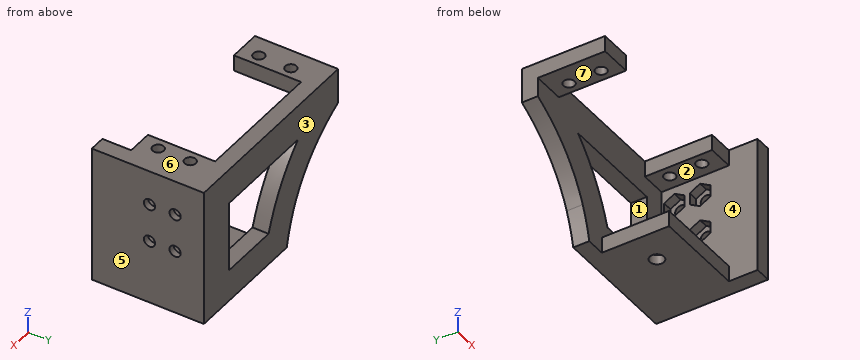
from build123d import *

# Parameters (mm, degrees)
SKETCH1_W                = 10
SKETCH1_H                = 5
BOSS_EXTRUDE1_DEPTH      = 21
BOSS_EXTRUDE1_2_DEPTH    = 21
SKETCH2_W                = 61
SKETCH2_H                = 43
BOSS_EXTRUDE2_DEPTH      = 5
SKETCH3_W                = 30.5
SKETCH3_H                = 5
BOSS_EXTRUDE3_DEPTH      = 21
CUT_EXTRUDE1_REACH       = 74.498
SKETCH4_R                = 2.2
CUT_EXTRUDE2_REACH       = 77.24
SKETCH5_R                = 1.75
CUT_EXTRUDE4_REACH       = 74.231
BOSS_EXTRUDE4_DEPTH      = 3
BOSS_EXTRUDE4_DEPTH_BACK = 2
SKETCH10_W               = 43
SKETCH10_H               = 35
CUT_EXTRUDE5_DEPTH       = 2
CUT_EXTRUDE6_REACH       = 82.077
SKETCH12_R               = 1.75
CUT_EXTRUDE7_DEPTH       = 3


with BuildPart() as part:
    # Sketch1 → Boss-Extrude1 (new body)
    with BuildSketch(Plane(origin=(0, 0, 0), x_dir=(1, 0, 0), z_dir=(0, 1, 0))):
        Rectangle(SKETCH1_W, SKETCH1_H)
    extrude(amount=BOSS_EXTRUDE1_DEPTH)



with BuildPart() as body_2:
    # Sketch1 → Boss-Extrude1 2 (new body)
    with BuildSketch(Plane(origin=(0, 0, 0), x_dir=(1, 0, 0), z_dir=(0, 1, 0))):
        with Locations((51, 0)):
            Rectangle(SKETCH1_W, SKETCH1_H)
    extrude(amount=BOSS_EXTRUDE1_2_DEPTH)


with BuildPart() as part_1:
    add(part.part)

    add(body_2.part)  # Boss-Extrude2 merges body 2
    # Sketch2 → Boss-Extrude2 (add)
    with BuildSketch(Plane(origin=(0, 21, 0), x_dir=(1, 0, 0), z_dir=(0, 1, 0))):
        with Locations((25.5, 19)):
            Rectangle(SKETCH2_W, SKETCH2_H)
    extrude(amount=BOSS_EXTRUDE2_DEPTH)

    # Sketch3 → Boss-Extrude3 (add)
    with BuildSketch(Plane.XZ.offset(-21)):
        with Locations((40.75, -38)):
            Rectangle(SKETCH3_W, SKETCH3_H)
    extrude(amount=BOSS_EXTRUDE3_DEPTH)

    # Sketch4 → Cut-Extrude1 (cut, up to next)
    with BuildSketch(Plane.XY.offset(-35.5), mode=Mode.PRIVATE) as cut_extrude1_sk1:
        with Locations((35.75, 10.5)):
            Circle(SKETCH4_R)
    cut_extrude1_tool1 = extrude(cut_extrude1_sk1.sketch, amount=-CUT_EXTRUDE1_REACH, mode=Mode.PRIVATE) & part_1.part
    add(cut_extrude1_tool1.solids().sort_by_distance((35.75, 10.5, -35.5))[0], mode=Mode.SUBTRACT)

    # Sketch5 → Cut-Extrude2 (cut, up to next)
    with BuildSketch(Plane.XY.offset(2.5), mode=Mode.PRIVATE) as cut_extrude2_sk1:
        with Locations((1.5, 15.5)):
            Circle(SKETCH5_R)
    cut_extrude2_tool1 = extrude(cut_extrude2_sk1.sketch, amount=-CUT_EXTRUDE2_REACH, mode=Mode.PRIVATE) & part_1.part
    # Sketch5 → Cut-Extrude2 (cut, up to next)
    with BuildSketch(Plane.XY.offset(2.5), mode=Mode.PRIVATE) as cut_extrude2_sk2:
        with Locations((49.5, 15.5)):
            Circle(SKETCH5_R)
    cut_extrude2_tool2 = extrude(cut_extrude2_sk2.sketch, amount=-CUT_EXTRUDE2_REACH, mode=Mode.PRIVATE) & part_1.part
    # Sketch5 → Cut-Extrude2 (cut, up to next)
    with BuildSketch(Plane.XY.offset(2.5), mode=Mode.PRIVATE) as cut_extrude2_sk3:
        with Locations((49.5, 5.5)):
            Circle(SKETCH5_R)
    cut_extrude2_tool3 = extrude(cut_extrude2_sk3.sketch, amount=-CUT_EXTRUDE2_REACH, mode=Mode.PRIVATE) & part_1.part
    # Sketch5 → Cut-Extrude2 (cut, up to next)
    with BuildSketch(Plane.XY.offset(2.5), mode=Mode.PRIVATE) as cut_extrude2_sk4:
        with Locations((1.5, 5.5)):
            Circle(SKETCH5_R)
    cut_extrude2_tool4 = extrude(cut_extrude2_sk4.sketch, amount=-CUT_EXTRUDE2_REACH, mode=Mode.PRIVATE) & part_1.part
    add(cut_extrude2_tool1.solids().sort_by_distance((1.5, 15.5, 2.5))[0], mode=Mode.SUBTRACT)
    add(cut_extrude2_tool2.solids().sort_by_distance((49.5, 15.5, 2.5))[0], mode=Mode.SUBTRACT)
    add(cut_extrude2_tool3.solids().sort_by_distance((49.5, 5.5, 2.5))[0], mode=Mode.SUBTRACT)
    add(cut_extrude2_tool4.solids().sort_by_distance((1.5, 5.5, 2.5))[0], mode=Mode.SUBTRACT)

    # Sketch7 → Cut-Extrude4 (cut, up to next)
    with BuildSketch(Plane.XZ.offset(-21), mode=Mode.PRIVATE) as cut_extrude4_sk1:
        with BuildLine():
            add(Edge.make_bspline(
                [(-5, -8.5), (10.13734929, -16.069431505), (16.393117595, -30.5)],
                knots=[0, 0, 0, 0.756510063, 0.756510063, 0.756510063], degree=2))
            Line((-5, -8.5), (-5, -40.5))
            Line((-5, -40.5), (19.5, -40.5))
            add(Edge.make_bspline(
                [(16.393117595, -30.5), (18.406595945, -35.144615311), (19.5, -40.5)],
                knots=[0.756510063, 0.756510063, 0.756510063, 1, 1, 1], degree=2))
        make_face()
    cut_extrude4_tool1 = extrude(cut_extrude4_sk1.sketch, amount=-CUT_EXTRUDE4_REACH, mode=Mode.PRIVATE) & part_1.part
    # Sketch7 → Cut-Extrude4 (cut, up to next)
    with BuildSketch(Plane.XZ.offset(-21), mode=Mode.PRIVATE) as cut_extrude4_sk2:
        with BuildLine():
            add(Edge.make_bspline(
                [(14.162446419, -8.5), (14.308605592, -8.637915777), (15.764925912, -10.027572407), (18.374354372, -12.814680355), (21.64995854, -17.12958205), (24.471025142, -21.768825406), (26.433850498, -25.877231684), (27.590424444, -28.831311595), (28.037332794, -30.099095454), (28.173885888, -30.5)],
                knots=[0.333258572, 0.333258572, 0.333258572, 0.333258572, 0.345023116, 0.45114151, 0.557259903, 0.663378297, 0.769496691, 0.822555887, 0.846906812, 0.846906812, 0.846906812, 0.846906812], degree=3))
            Line((28.173885888, -30.5), (47, -30.5))
            Line((47, -30.5), (47, -8.5))
            Line((47, -8.5), (46, -8.5))
            Line((46, -8.5), (14.162446419, -8.5))
        make_face()
    cut_extrude4_tool2 = extrude(cut_extrude4_sk2.sketch, amount=-CUT_EXTRUDE4_REACH, mode=Mode.PRIVATE) & part_1.part
    add(cut_extrude4_tool1.solids().sort_by_distance((4.583978, 21, -28.190426))[0], mode=Mode.SUBTRACT)
    add(cut_extrude4_tool2.solids().sort_by_distance((34.394415, 21, -18.474006))[0], mode=Mode.SUBTRACT)

    # Sketch10 → Boss-Extrude4 (add, two sides: drawn at the far end of the back side and taken through both)
    with BuildSketch(Plane(origin=(56, 0, 0), x_dir=(0, 0, -1), z_dir=(1, 0, 0)).offset(-BOSS_EXTRUDE4_DEPTH_BACK)):
        with Locations((19, 8.5)):
            Rectangle(SKETCH10_W, SKETCH10_H)
    extrude(amount=BOSS_EXTRUDE4_DEPTH + BOSS_EXTRUDE4_DEPTH_BACK)

    # Sketch11 → Cut-Extrude5 (cut)
    with BuildSketch(Plane.XY.offset(-35.5)):
        Polygon((37.886195996, 14.2), (33.613804004, 14.2), (31.477608008, 10.5), (33.613804004, 6.8), (37.886195996, 6.8), (40.022391992, 10.5), align=None)
    extrude(amount=-CUT_EXTRUDE5_DEPTH, mode=Mode.SUBTRACT)

    # Sketch12 → Cut-Extrude6 (cut, up to next)
    with BuildSketch(Plane(origin=(59, 0, 0), x_dir=(0, 0, -1), z_dir=(1, 0, 0)), mode=Mode.PRIVATE) as cut_extrude6_sk1:
        with Locations((8.4, 17)):
            Circle(SKETCH12_R)
    cut_extrude6_tool1 = extrude(cut_extrude6_sk1.sketch, amount=-CUT_EXTRUDE6_REACH, mode=Mode.PRIVATE) & part_1.part
    # Sketch12 → Cut-Extrude6 (cut, up to next)
    with BuildSketch(Plane(origin=(59, 0, 0), x_dir=(0, 0, -1), z_dir=(1, 0, 0)), mode=Mode.PRIVATE) as cut_extrude6_sk2:
        with Locations((8.4, 9)):
            Circle(SKETCH12_R)
    cut_extrude6_tool2 = extrude(cut_extrude6_sk2.sketch, amount=-CUT_EXTRUDE6_REACH, mode=Mode.PRIVATE) & part_1.part
    # Sketch12 → Cut-Extrude6 (cut, up to next)
    with BuildSketch(Plane(origin=(59, 0, 0), x_dir=(0, 0, -1), z_dir=(1, 0, 0)), mode=Mode.PRIVATE) as cut_extrude6_sk3:
        with Locations((20.4, 17)):
            Circle(SKETCH12_R)
    cut_extrude6_tool3 = extrude(cut_extrude6_sk3.sketch, amount=-CUT_EXTRUDE6_REACH, mode=Mode.PRIVATE) & part_1.part
    # Sketch12 → Cut-Extrude6 (cut, up to next)
    with BuildSketch(Plane(origin=(59, 0, 0), x_dir=(0, 0, -1), z_dir=(1, 0, 0)), mode=Mode.PRIVATE) as cut_extrude6_sk4:
        with Locations((20.4, 9)):
            Circle(SKETCH12_R)
    cut_extrude6_tool4 = extrude(cut_extrude6_sk4.sketch, amount=-CUT_EXTRUDE6_REACH, mode=Mode.PRIVATE) & part_1.part
    add(cut_extrude6_tool1.solids().sort_by_distance((59, 17, -8.4))[0], mode=Mode.SUBTRACT)
    add(cut_extrude6_tool2.solids().sort_by_distance((59, 9, -8.4))[0], mode=Mode.SUBTRACT)
    add(cut_extrude6_tool3.solids().sort_by_distance((59, 17, -20.4))[0], mode=Mode.SUBTRACT)
    add(cut_extrude6_tool4.solids().sort_by_distance((59, 9, -20.4))[0], mode=Mode.SUBTRACT)

    # Sketch13 → Cut-Extrude7 (cut)
    with BuildSketch(Plane.ZY.offset(-54)):
        Polygon((-12.095041723, 17), (-10.247520861, 13.8), (-6.552479139, 13.8), (-4.704958277, 17), (-6.552479139, 20.2), (-10.247520861, 20.2), align=None)
        Polygon((-10.247520861, 5.8), (-6.552479139, 5.8), (-4.704958277, 9), (-6.552479139, 12.2), (-10.247520861, 12.2), (-12.095041723, 9), align=None)
        Polygon((-18.552479139, 20.2), (-22.247520861, 20.2), (-24.095041723, 17), (-22.247520861, 13.8), (-18.552479139, 13.8), (-16.704958277, 17), align=None)
        Polygon((-22.247520861, 12.2), (-24.095041723, 9), (-22.247520861, 5.8), (-18.552479139, 5.8), (-16.704958277, 9), (-18.552479139, 12.2), align=None)
    extrude(amount=-CUT_EXTRUDE7_DEPTH, mode=Mode.SUBTRACT)


solid = part_1.part
Geometry check sheet. Reference: the model listing, model coordinates, mm. Face numbers are marked on the shaded views. A direction names the side the tool comes from. Round coordinates to 2 decimals unless told otherwise and drop trailing zeros. Loops run counter-clockwise (first coordinate to the right, second up) from the corner with the lowest first, then second, coordinate; pieces in that order, holes last.
Item 1: Cross-section at B-B on z = 0. Record the boundary of the cut face in (x, y), then the cut area to 3 significant figures.
Item 2: Gauge pin test, flat ends, axial feed: pin 1 (5 mm diameter, centred on x = 35.75, y = 10.5, fed in from +Z); pin 2 (3 mm diameter, centred on x = 14, z = -28, fed in from -Y); pin 3 (4 mm diameter, centred on x = 37, z = -37, fed in from -Y); pin 4 (4.5 mm diameter, centred on x = 1.5, y = 15.5, fed in from +Z). Record the tip position at first contact, or that the pin passes through.
Item 3: Cross-section at D-D on x = 49.5. Record the boundary of the cut face in (y, z).
Item 4: Thickness scan on line 1 (Y direction, x = 1.5, z = 1.5); line 2 (Y direction, x = 58.6, z = -20.4); line 3 (Z direction, x = 34.5, y = 23.5). Record the ranges inside material, lowest first.
Item 5: Access from +Z, -Z, +X, -X, +Y, -Y to the whole of each face (thin tool, end or side, straight path). Record for the marked faces 1, 2 and 3.
Item 6: Mould release check, pull along Z, two halves, no side actions. Record for the marked faces 4, 5, 6 and 7: pulls with the +Z half, pulls with the -Z half, needs draft (parallel to the pull), parting line crosses it, or undercut.
Item 7: Cross-section at C-C on z = -7.5. Record the boundary of the cut face in (x, y).
Item 8: Cross-section at A-A on x = 35.75. Record the boundary of the cut face in (y, z).
Answer sheet:
1. outline: (-5, 0) - (5, 0) - (5, 21) - (46, 21) - (46, 0) - (54, 0) - (54, -9) - (59, -9) - (59, 26) - (-5, 26) - close; hole circle Ø3.5 at (1.5, 5.5); hole circle Ø3.5 at (1.5, 15.5); hole circle Ø3.5 at (49.5, 5.5); hole circle Ø3.5 at (49.5, 15.5)
1. area: 810 mm2
2. pin 1: stops at z = -37.5
2. pin 2: stops at y = 21
2. pin 3: stops at y = 0
2. pin 4: stops at z = 2.5
3. outline: (0, -40.5) - (26, -40.5) - (26, 2.5) - (17.25, 2.5) - (17.25, -2.5) - (21, -2.5) - (21, -35.5) - (0, -35.5) - close; (0, -2.5) - (3.75, -2.5) - (3.75, 2.5) - (0, 2.5) - close; (7.25, -2.5) - (13.75, -2.5) - (13.75, 2.5) - (7.25, 2.5) - close
4. line 1: y = 0 to 3.75, 7.25 to 13.75, 17.25 to 26
4. line 2: y = -9 to 7.25, 10.75 to 15.25, 18.75 to 26
4. line 3: z = -40.5 to -30.5, -8.5 to 2.5
5. face 1: +Y, -Y
5. face 2: -X, -Y
5. face 3: +Z, -Z, +X, -X, +Y
6. face 4: undercut
6. face 5: needs draft
6. face 6: pulls with the +Z half
6. face 7: pulls with the -Z half
7. outline: (-5, 21) - (54, 21) - (54, 20.2) - (57, 20.2) - (57, 18.5) - (59, 18.5) - (59, 26) - (-5, 26) - close; (54, -9) - (59, -9) - (59, 7.5) - (57, 7.5) - (57, 5.8) - (54, 5.8) - close; (54, 12.2) - (57, 12.2) - (57, 10.5) - (59, 10.5) - (59, 15.5) - (57, 15.5) - (57, 13.8) - (54, 13.8) - close
8. outline: (0, -40.5) - (8.3, -40.5) - (8.3, -37.5) - (6.8, -37.5) - (6.8, -35.5) - (0, -35.5) - close; (12.7, -40.5) - (26, -40.5) - (26, -30.5) - (21, -30.5) - (21, -35.5) - (14.2, -35.5) - (14.2, -37.5) - (12.7, -37.5) - close; (21, -8.5) - (26, -8.5) - (26, 2.5) - (21, 2.5) - close
